Source: CAD feature listing. Evaluate the final solid. Frame: model axes, mm. A direction names the side the tool comes from. Round coordinates to 2 decimals unless told otherwise and drop trailing zeros. Write each loop counter-clockwise with the first axis right and the second up, starting at its lowest first coordinate (ties: lowest second). Pieces come first, ordered by that corner, then holes.
from build123d import *

# Parameters (mm, degrees)
FILLET1_R   = 0.25
FILLET2_R   = 0.3
HEX_2_DEPTH = 3


with BuildPart() as part:
    # BodySke → Base-Revolve (revolve)
    with BuildSketch(Plane.XY, mode=Mode.PRIVATE) as base_revolve_sk:
        Polygon((0, 0), (0, 5), (6, 5), (6, 3), (30.4455, 3), (31, 2.4455), (31, 0), align=None)
    revolve(base_revolve_sk.sketch.rotate(Axis((-31.75, 0, 0), (1, 0, 0)), 90), axis=Axis((-31.75, 0, 0), (1, 0, 0)))  # turned: the seam where the file's is

    # Fillet1
    fillet1_edges = [part.edges().sort_by_distance(p)[0] for p in [
        (6, 0, -3),
    ]]
    fillet(fillet1_edges, radius=FILLET1_R)

    # Fillet2
    fillet2_edges = [part.edges().sort_by_distance(p)[0] for p in [
        (0, 0, -5),
    ]]
    fillet(fillet2_edges, radius=FILLET2_R)

    # Sketch2 → Hex-PreBroach (revolve, cut)
    with BuildSketch(Plane.XY, mode=Mode.PRIVATE) as hex_prebroach_sk:
        Polygon((0, 2.542), (3, 2.542), (4.467624384, 0), (0, 0), align=None)
    revolve(hex_prebroach_sk.sketch.rotate(Axis((0, 0, 0), (1, 0, 0)), 90), axis=Axis((0, 0, 0), (1, 0, 0)), mode=Mode.SUBTRACT)  # turned: the seam where the file's is

    # Sketch3 → Hex 2 (cut)
    with BuildSketch(Plane(origin=(0, 0, 0), x_dir=(0, 0.5, 0.866025404), z_dir=(-1, 0, 0))):
        Polygon((1.467624384, 2.542), (-1.467624384, 2.542), (-2.935248769, 0), (-1.467624384, -2.542), (1.467624384, -2.542), (2.935248769, 0), align=None)
    extrude(amount=-HEX_2_DEPTH, mode=Mode.SUBTRACT)


solid = part.part
1) Contact query for flat-ended pins moving along their axis: P1, Ø4, axis at x = 19.5, z = -1, coming from the -Y side; P2, Ø2, axis at y = 4, z = -1, coming from the +X side; P3, Ø2, axis at x = 16.5, y = -3, coming from the +Z side. Output: stop coordinate, or through.
Taken from the geometry:
P1: stops at y = -3
P2: stops at x = 6.03
P3: stops at z = 2.24
2) Section query A-A on x = 7.5. Return the cut outline in (y, z), then the cut area to 3 significant figures.
Taken from the geometry:
outline: circle Ø6 at (0, 0)
area: 28.3 mm2
3) Reachability of faces 1 (the face through (0, 2, -2)), 2 (the face through (3, 1.4, -2.3)), 3 (the face through (6, 1, 3.3)) from +Z, -Z, +X, -X, +Y, -Y: full face, straight path, thin tool, end or side. Return the list, or none.
Taken from the geometry:
face 1: +Z, -Z, -X, +Y, -Y
face 2: -X
face 3: +X
4) Pull-direction query (Z, two-part tool) for faces 4 (the face through (31, 0, 0)), 5 (the face through (18.52, -0.9, 2.86)), 6 (the face through (4.233, 0.247, -0.322)); classes: released by +Z, released by -Z, zero draft, split by the parting line, or undercut.
Taken from the geometry:
face 4: zero draft
face 5: split by the parting line
face 6: undercut
5) Material intervals for line 1 (X direction, y = 3.25, z = -2.75); line 2 (Y direction, x = 2, z = -4); line 3 (X direction, y = -1.75, z = -2.5), sorted ascending.
Taken from the geometry:
line 1: x = 0 to 6
line 2: y = -3 to 3
line 3: x = 0 to 6.1
